Can you work these out from the model? Positions are in its coordinate system, mm. A direction names the side the tool comes from. Coordinates: 2 decimals unless noted, no trailing zeros. Order: outer loops, then holes, each group sorted by start corner. A loop starts at its lowest first (then second) coordinate and runs counter-clockwise, first axis right, second up.
```python
from build123d import *

# Parameters (mm, degrees)
F0_R     = 152.4
F0_R_2   = 12.7
F1_DEPTH = 6.35


with BuildPart() as f1:
    # F0 (on Top) → F1 (new body)
    with BuildSketch(Plane.XY):
        Circle(F0_R)
        with BuildLine():
            ThreePointArc((-50.8, -116.813009), (-127.381, 0), (-50.8, 116.813009))
            Line((-50.8, 116.813009), (-50.8, 94.817982))
            ThreePointArc((-50.8, 94.817982), (-107.569, 0), (-50.8, -94.817982))
            Line((-50.8, -94.817982), (-50.8, -116.813009))
        make_face(mode=Mode.SUBTRACT)
        Circle(F0_R_2, mode=Mode.SUBTRACT)
        with BuildLine():
            Line((50.8, 94.817982), (50.8, 116.813009))
            ThreePointArc((50.8, 116.813009), (127.381, 0), (50.8, -116.813009))
            Line((50.8, -116.813009), (50.8, -94.817982))
            ThreePointArc((50.8, -94.817982), (107.569, 0), (50.8, 94.817982))
        make_face(mode=Mode.SUBTRACT)
    extrude(amount=F1_DEPTH)


solid = f1.part
```
1. On a 3-axis mill with a long thin cutter (end or side, diameter ignored), from which of +Z, -Z, +X, -X, +Y, -Y can I reach the whole of each face in a straight line? I mean faces 1 (the flat face through (32, 2, 6.35)), 2 (the cylindrical face through (-107.557, 1.625, 3.131)). Say none if no direction works.
Completed:
face 1: +Z, +X, -X, +Y, -Y
face 2: +Z, -Z
2. Thinking about a two-plate mould opening in Y: for faces 3 (the cylindrical face through (127.364, 2.07, 3.131)), 4 (the cylindrical face through (-120.94, -92.73, 3.13)), 5 (the flat face through (32, 2, 0)), which applies, pulls with the +Y half, pulls with the -Y half, needs draft (parallel to the pull), parting line crosses it, or undercut?
Completed:
face 3: undercut
face 4: parting line crosses it
face 5: needs draft
3. Please list where these lines run through material, in increasing order: probe 1 along Y at (x, z) = (0, 3.25); probe 2 along Y at (x, z) = (94.5, 5.5); probe 3 along X at (y, z) = (74, 5.5).
Completed:
probe 1: y = -152.4 to -12.7, 12.7 to 152.4
probe 2: y = -119.56 to -85.41, -51.39 to 51.39, 85.41 to 119.56
probe 3: x = -133.23 to -103.68, -78.07 to 78.07, 103.68 to 133.23
4. Imagine slicing it at D-D on y = 54.5. Please give me the cut outline in (x, z).
Completed:
outline: (-142.32, 0) - (-115.13, 0) - (-115.13, 6.35) - (-142.32, 6.35) - close; (-92.74, 0) - (92.74, 0) - (92.74, 6.35) - (-92.74, 6.35) - close; (115.13, 0) - (142.32, 0) - (142.32, 6.35) - (115.13, 6.35) - close
5. I'm going to push flat-ended pins straight in: pin 1 (1 mm diameter, centred on x = -79, z = 2, fed in from -Y); pin 2 (20.5 mm diameter, centred on x = 0, y = 0, fed in from -Z); pin 3 (2 mm diameter, centred on x = 21.5, z = 3, fed in from +Y); pin 4 (2 mm diameter, centred on y = 30.5, z = 1, fed in from +X). Where does each tip first touch, or does it pass through?
Completed:
pin 1: stops at y = -130.63
pin 2: passes through
pin 3: stops at y = 151.01
pin 4: stops at x = 149.52
6. Imagine slicing it at A-A on x = 0. Please give me the cut outline in (y, z).
Completed:
outline: (-152.4, 0) - (-12.7, 0) - (-12.7, 6.35) - (-152.4, 6.35) - close; (12.7, 0) - (152.4, 0) - (152.4, 6.35) - (12.7, 6.35) - close
7. Imagine slicing it at B-B on y = 0. Please give me the cut outline in (x, z), then the cut area to 3 significant figures.
Completed:
outline: (-152.4, 0) - (-127.38, 0) - (-127.38, 6.35) - (-152.4, 6.35) - close; (-107.57, 0) - (-12.7, 0) - (-12.7, 6.35) - (-107.57, 6.35) - close; (12.7, 0) - (107.57, 0) - (107.57, 6.35) - (12.7, 6.35) - close; (127.38, 0) - (152.4, 0) - (152.4, 6.35) - (127.38, 6.35) - close
area: 1,520 mm2
8. Imagine slicing it at C-C on z = 3.75. Please give me the cut outline in (x, y), then the cut area to 3 significant figures.
Completed:
outline: circle Ø304.8 at (0, 0); hole (-50.8, -116.81) - (-50.8, -94.82) arc R107.57 cw to (-50.8, 94.82) - (-50.8, 116.81) arc R127.38 ccw to start; hole circle Ø25.4 at (0, 0); hole (50.8, -116.81) arc R127.38 ccw to (50.8, 116.81) - (50.8, 94.82) arc R107.57 cw to (50.8, -94.82) - close
area: 62,000 mm2
